Check sheet for the modelled part. Datum: model origin and axes. Units: mm. A direction names the side the tool comes from. Coordinates: 2 decimals unless noted, no trailing zeros. Loops run counter-clockwise (first coordinate to the right, second up) from the corner with the lowest first, then second, coordinate; pieces in that order, holes last.
```python
from build123d import *

# Parameters (mm, degrees)
SKETCH1_W           = 144
SKETCH1_H           = 64
BOSS_EXTRUDE1_DEPTH = 16
BOSS_EXTRUDE2_DEPTH = 64
SKETCH3_R           = 8
BOSS_EXTRUDE3_DEPTH = 22
FILLET1_R           = 2
CUT_EXTRUDE1_DEPTH  = 157.409718368


with BuildPart() as part:
    # Sketch1 → Boss-Extrude1 (new body)
    with BuildSketch(Plane(origin=(0, 0, 0), x_dir=(1, 0, 0), z_dir=(0, 1, 0))):
        Rectangle(SKETCH1_W, SKETCH1_H)
    extrude(amount=BOSS_EXTRUDE1_DEPTH)

    # Sketch2 → Boss-Extrude2 (add)
    with BuildSketch(Plane.XY.offset(32)):
        Polygon((-72, 16), (-72, 38), (-56, 52), (-46, 52), (-46, 16), align=None)
    extrude(amount=-BOSS_EXTRUDE2_DEPTH)

    # Sketch3 → Boss-Extrude3 (add)
    with BuildSketch(Plane(origin=(72, 0, 0), x_dir=(0, 0, -1), z_dir=(1, 0, 0))):
        with BuildLine():
            Line((-27.556282819, 16), (-14.380704741, 43.013938349))
            ThreePointArc((-14.380704741, 43.013938349), (0, 52), (14.380704741, 43.013938349))
            Line((14.380704741, 43.013938349), (27.556282819, 16))
            Line((27.556282819, 16), (-27.556282819, 16))
        make_face()
        with Locations((0, 36)):
            Circle(SKETCH3_R, mode=Mode.SUBTRACT)
    extrude(amount=-BOSS_EXTRUDE3_DEPTH)

    # Fillet1
    fillet1_edges = [part.edges().sort_by_distance(p)[0] for p in [
        (61, 16, -27.556282819),
        (61, 16, 27.556282819),
    ]]
    fillet(fillet1_edges, radius=FILLET1_R)

    # Sketch4 → Cut-Extrude1 (cut, through all)
    with BuildSketch(Plane(origin=(72, 0, 0), x_dir=(0, 0, -1), z_dir=(1, 0, 0))):
        Polygon((-16, 0), (-16, 7), (-8, 7), (-8, 16), (8, 16), (8, 7), (16, 7), (16, 0), align=None)
    extrude(amount=-CUT_EXTRUDE1_DEPTH, mode=Mode.SUBTRACT)


solid = part.part
```
1) Section check C-C on x = 14. Enter the section's corners in (y, z), plus the area to 3 significant figures.
Answer sheet:
outline: (0, -32) - (16, -32) - (16, -8) - (7, -8) - (7, -16) - (0, -16) - close; (0, 16) - (7, 16) - (7, 8) - (16, 8) - (16, 32) - (0, 32) - close
area: 656 mm2
2) Mould release check, pull along Z, two halves, no side actions. Record for faces 5 (the cylindrical face through (61, 52, 0)), 6 (the flat face through (72, 20, 0)), 7 (the flat face through (1, 3, 16)): +Z half, -Z half, draft (parallel to the pull), parting line (faces both ways), or undercut.
Answer sheet:
face 5: parting line
face 6: draft
face 7: undercut
3) Section check D-D on x = -52.5. Enter the section's corners in (y, z), plus the area to 3 significant figures.
Answer sheet:
outline: (0, -32) - (52, -32) - (52, 32) - (0, 32) - (0, 16) - (7, 16) - (7, 8) - (16, 8) - (16, -8) - (7, -8) - (7, -16) - (0, -16) - close
area: 2,960 mm2
4) Set-up check for faces 1 (the flat face through (61.154, 30.25, -20.606)), 2 (the flat face through (61.15, 29.89, 20.78)), 3 (the flat face through (1, 12, -8)), 4 (the cylindrical face through (61.154, 43.932, 1.041)): record each of +Z, -Z, +X, -X, +Y, -Y from which the full face is reachable in a straight line by a thin tool's end or side.
Answer sheet:
face 1: -Z, +X, +Y
face 2: +Z, +X, +Y
face 3: +X, -X, -Y
face 4: +X
5) Section check B-B on y = 5. Enter the section's corners in (x, z).
Answer sheet:
outline: (-72, -32) - (72, -32) - (72, -16) - (-72, -16) - close; (-72, 16) - (72, 16) - (72, 32) - (-72, 32) - close
6) Scan lines: line 1 (X direction, y = 29, z = 8); line 2 (Y direction, x = 62, z = 0); line 3 (Y direction, x = -3, z = -26). Record each from-to range of solid material in increasing order.
Answer sheet:
line 1: x = -72 to -46, 50 to 72
line 2: y = 16 to 28, 44 to 52
line 3: y = 0 to 16
7) Depth check by flat-ended pin: pin 1 (12 mm diameter, centred on x = -5, z = -21, fed in from +Y); pin 2 (4 mm diameter, centred on x = 33, z = 12, fed in from -Y); pin 3 (13 mm diameter, centred on x = -59, z = 1, fed in from -Y). Enter the tip coordinate at first touch or a pass-through.
Answer sheet:
pin 1: stops at y = 16
pin 2: stops at y = 7
pin 3: stops at y = 16
8) Section check A-A on z = 0. Enter the section's corners in (x, y).
Answer sheet:
outline: (-72, 16) - (-46, 16) - (-46, 52) - (-56, 52) - (-72, 38) - close; (50, 16) - (72, 16) - (72, 28) - (50, 28) - close; (50, 44) - (72, 44) - (72, 52) - (50, 52) - close
